Autodesk Inventor part; units mm, degrees
ref_plane "РабПлоскость2" through (-11.5, 28.8975, 52.6492) normal (0, 0, -1) x (0, 1, 0)
ref_plane "РабПлоскость3" through (-11.5, 28.8975, 52.6492) normal (0, 0, -1) x (0, 1, 0)
ref_plane "РабПлоскость4" through (-15, 28.8975, 52.6492) normal (0, -1, 0) x (1, 0, 0)
ref_plane "РабПлоскость1" through (0, 34.8975, 74.4992) normal (0, 0, -1) x (1, 0, 0)
sketch "Эскиз1" plane through (0, 34.8975, 74.4992) normal (0, 0, -1) x (1, 0, 0)
  line L0 (11.5, 6) -> (11.5, -6)
  line L1 (15, -6) -> (11.5, -6)
  arc A0 (15, -6) -> (16, -5) centre (15, -5) ccw
  line L2 (16, -1.25) -> (16, -5)
  line L3 (14, -1.25) -> (16, -1.25)
  arc A1 (12.8, -0.05) -> (14, -1.25) centre (14, -0.05) ccw
  line L4 (12.8, 0.05) -> (12.8, -0.05)
  arc A2 (14, 1.25) -> (12.8, 0.05) centre (14, 0.05) ccw
  line L5 (16, 1.25) -> (14, 1.25)
  line L6 (16, 5) -> (16, 1.25)
  arc A3 (16, 5) -> (15, 6) centre (15, 5) ccw
  line L7 (11.5, 6) -> (15, 6)
  circle A4 centre (13.75, 3.5) radius 1.25
  circle A5 centre (13.75, -3.5) radius 1.25
  line L8 (-11.5, -6) -> (-11.5, 6)
  line L9 (-15, 6) -> (-11.5, 6)
  arc A6 (-15, 6) -> (-16, 5) centre (-15, 5) ccw
  line L10 (-16, 1.3872) -> (-16, 5)
  line L11 (-14, 1.3872) -> (-16, 1.3872)
  arc A7 (-12.802, 0.1186) -> (-14, 1.3872) centre (-14, 0.1872) ccw
  line L12 (-12.802, 0.0186) -> (-12.802, 0.1186)
  arc A8 (-14, -1.25) -> (-12.802, 0.0186) centre (-14, -0.05) ccw
  line L13 (-16, -1.25) -> (-14, -1.25)
  line L14 (-16, -5) -> (-16, -1.25)
  arc A9 (-16, -5) -> (-15, -6) centre (-15, -5) ccw
  line L15 (-11.5, -6) -> (-15, -6)
  circle A10 centre (-13.75, 3.5) radius 1.25
  circle A11 centre (-13.75, -3.5) radius 1.25
  line L16 (16, 5) -> (16, 6)
  line L17 (16, 6) -> (15, 6)
  line L18 (-16, 5) -> (-16, 6)
  line L19 (-16, 6) -> (-15, 6)
  line L20 (16, -5) -> (16, -6)
  line L21 (16, -6) -> (15, -6)
  line L22 (-16, -5) -> (-16, -6)
  line L23 (-16, -6) -> (-15, -6)
  point P0 (0, 34.8975)
extrude "Выдавливание1" add sketch "Эскиз1" along normal blind 6
sketch "Эскиз3" plane through (11.5, 28.8975, 74.4992) normal (0, -1, 0) x (1, 0, 0)
  line L0 (-23, 0) -> (-23, -6)
  line L1 (-23, -6) -> (-23, 0)
  line L2 (-23, 0) -> (-27.5, 0)
  line L3 (0, -6) -> (-23, -6)
  line L4 (-23, -6) -> (-23, 0)
  line L5 (-23, 0) -> (0, 0)
  line L6 (-23, -6) -> (-27.5, -6)
  line L7 (-23, -6) -> (-27.5, -6)
  line L8 (-27.5, -6) -> (-27.5, 0)
  line L9 (0, 0) -> (4.5, 0)
  line L10 (0, -6) -> (0, 0)
  line L11 (4.5, 0) -> (4.5, -6)
  line L12 (4.5, -6) -> (0, -6)
  point P0 (-11.5, -74.4992)
  point P1 (4.5, 0)
extrude "Выдавливание2" add sketch "Эскиз3" along normal blind 30
ref_plane "РабПлоскость2" through (-11.5, 28.8975, 52.6492) normal (0, 0, -1) x (0, 1, 0)
ref_plane "РабПлоскость3" through (-11.5, 28.8975, 52.6492) normal (0, 0, -1) x (0, 1, 0)
ref_plane "РабПлоскость6" through (-16, 2.8975, 68.4992) normal (0, 1, 0) x (1, 0, 0)
ref_plane "РабПлоскость4" through (-15, 28.8975, 52.6492) normal (0, -1, 0) x (1, 0, 0)
ref_plane "РабПлоскость8" through (-16, 2.8975, 68.4992) normal (0, 1, 0) x (1, 0, 0)
ref_plane "РабПлоскость5" through (-16, 2.8975, 68.4992) normal (0, 1, 0) x (1, 0, 0)
ref_plane "РабПлоскость7" through (16, 28.8975, 74.4992) normal (1, 0, 0) x (0, 0, -1)
ref_plane "РабПлоскость9" through (16, 28.8975, 74.4992) normal (-1, 0, 0) x (0, 0, 1)
ref_plane "РабПлоскость10" through (-16, 28.8975, 74.4992) normal (-1, 0, 0) x (0, 0, 1)
sketch "Эскиз14" plane through (11.5, -1.1025, 74.4992) normal (0, -1, 0) x (1, 0, 0)
  circle A0 centre (-3.5, -11.925) radius 2
  circle A1 centre (-19.5, -11.925) radius 2
  circle A2 centre (-3.5, -11.925) radius 1.5
  circle A3 centre (-19.5, -11.925) radius 1.5
  point P0 (-11.5, -74.4992)
  dimension "d38" = 3
  dimension "d39" = 3
extrude "Выдавливание12" add sketch "Эскиз14" against normal blind 4
ref_plane "РабПлоскость14" through (18, 28.8975, 74.4992) normal (1, 0, 0) x (0, 0, -1)
sketch "Эскиз15" plane through (18, 28.8975, 74.4992) normal (1, 0, 0) x (0, 0, -1)
  line L0 (1.45, -3.75) -> (1.45, -63.75)
  line L1 (-2.55, -3.75) -> (1.45, -3.75)
  line L2 (-2.55, -3.75) -> (1.45, -3.75)
  line L3 (1.45, -3.75) -> (1.45, -34.5952)
  line L4 (1.45, -34.5952) -> (-2.55, -34.5952)
  line L5 (-2.55, -34.5952) -> (-2.55, -3.75)
  point P0 (74.4992, -28.8975)
extrude "Выдавливание13" cut sketch "Эскиз15" against normal blind 100
ref_plane "РабПлоскость13" through (16, 2.8975, 68.4992) normal (0, 1, 0) x (1, 0, 0)
ref_plane "РабПлоскость12" through (-18, 28.8975, 74.4992) normal (-1, 0, 0) x (0, 0, 1)
ref_plane "РабПлоскость11" through (16, 28.8975, 52.6492) normal (0, 0, -1) x (-1, 0, 0)
sketch "Эскиз18" plane through (16, 28.8975, 52.6492) normal (0, 0, -1) x (-1, 0, 0)
  circle A0 centre (4, -6.8) radius 1.5
  circle A1 centre (28, -6.8) radius 1.5
  point P0 (16, -28.8975)
extrude "Выдавливание16" cut sketch "Эскиз18" along normal mid plane 73
sketch "Эскиз19" plane through (0, 34.8975, 68.4992) normal (0, 0, -1) x (-1, 0, 0)
  line L0 (-16, -36) -> (16, -36)
  line L1 (16, -1.3872) -> (16, -36)
  line L2 (-16, -36) -> (16, -36)
  line L3 (16, -36) -> (16, -16)
  line L4 (16, -16) -> (-16, -16)
  line L5 (-16, -16) -> (-16, -36)
  point P0 (0, -34.8975)
  point P1 (11.5, -36)
  point P2 (16, -36)
  dimension "d57" = 20
extrude "Выдавливание17" cut sketch "Эскиз19" along normal mid plane 200
sketch "Эскиз13" plane through (-16, 28.8975, 74.4992) normal (-1, 0, 0) x (0, 0, 1)
  line L0 (-21.85, 12) -> (0, 12)
  line L1 (0, 12) -> (0, -10)
  line L2 (0, -10) -> (-21.85, -10)
  line L3 (-21.85, -10) -> (-21.85, 12)
  line L4 (0, 4.6128) -> (0, -3.75)
  point P0 (-74.4992, -28.8975)
  point P1 (0, 12)
  point P2 (-21.85, -30)
  dimension "d60" = 21.85
  dimension "d61" = 22
  dimension "d62" = 0
sketch "Эскиз10" plane through (16, 28.8975, 74.4992) normal (1, 0, 0) x (0, 0, -1)
  line L0 (0, 12) -> (21.85, 12)
  line L1 (21.85, 12) -> (21.85, -10)
  line L2 (21.85, -10) -> (0, -10)
  line L3 (0, -10) -> (0, 12)
  line L4 (0, 12) -> (6, 12)
  line L5 (0, 4.75) -> (0, -3.75)
  point P0 (74.4992, -28.8975)
  point P1 (21.85, -30)
  dimension "d63" = 21.85
  dimension "d64" = 22
  dimension "d65" = 0
  dimension "d66" = 0
extrude "Выдавливание18" add sketch "Эскиз13" along normal blind 2
extrude "Выдавливание19" add sketch "Эскиз10" along normal blind 2
sketch "Эскиз20" plane through (-16, 18.8975, 52.6492) normal (0, -1, 0) x (1, 0, 0)
  line L0 (32, 4) -> (0, 4)
  line L1 (0, 4) -> (0, 15.85)
  line L2 (0, 15.85) -> (32, 15.85)
  line L3 (32, 15.85) -> (32, 4)
  line L4 (0, 0) -> (0, 15.85)
  line L5 (32, 15.85) -> (0, 15.85)
  circle A0 centre (24, 9.925) radius 1.5
  circle A1 centre (8, 9.925) radius 1.5
  point P0 (16, -52.6492)
  dimension "d71" = 32
  dimension "d72" = 11.85
  dimension "d73" = 0
  dimension "d74" = 0
  dimension "d75" = 3
  dimension "d76" = 3
  dimension "d77" = 8
  dimension "d78" = 8
  dimension "d79" = 5.925
  dimension "d80" = 5.925
extrude "Выдавливание20" add sketch "Эскиз20" against normal blind 8.75
sketch "Эскиз21" plane through (16, 28.8975, 74.4992) normal (-1, 0, 0) x (0, 0, 1)
  line L0 (-21.85, 12) -> (-17.85, 12)
  line L1 (-17.85, 12) -> (-17.85, -10)
  line L2 (-17.85, -10) -> (-21.85, -10)
  line L3 (-21.85, -10) -> (-21.85, 12)
  line L4 (-17.85, -10) -> (-21.85, -10)
  line L5 (-17.85, -10) -> (-17.85, -1.25)
  point P0 (-74.4992, -28.8975)
  point P1 (-19.85, -10)
  dimension "d83" = 4
  dimension "d84" = 22
  dimension "d85" = 0
  dimension "d86" = 0
extrude "Выдавливание21" add sketch "Эскиз21" along normal blind 32.5
sketch "Эскиз22" plane through (-18, 18.8975, 52.6492) normal (0, 0, -1) x (-1, 0, 0)
  line L0 (-29.5, 10) -> (-29.5, 22)
  line L1 (-6.5, 22) -> (-6.5, 10)
  line L2 (-29.5, 10) -> (-6.5, 10)
  line L3 (-6.5, 10) -> (-6.5, 22)
  line L4 (-6.5, 22) -> (-29.5, 22)
  line L5 (-29.5, 22) -> (-29.5, 10)
  point P0 (-18, -18.8975)
extrude "Выдавливание22" cut sketch "Эскиз22" against normal blind 32.5
chamfer "Фаска1" distance 2 angle 45 2 edges at (6.5, 27.6475, 62.5742) (-9.5, 27.6475, 62.5742)
properties part number "держатель сервомоторчика"
Geometry: final body of the model. Coordinates: model frame, mm. A direction names the side the tool comes from. Round coordinates to 2 decimals unless told otherwise and drop trailing zeros. Write each loop counter-clockwise with the first axis right and the second up, starting at its lowest first coordinate (ties: lowest second). Pieces come first, ordered by that corner, then holes. Notation, with made-up numbers: M 40,-13.5 L 95,-13.5 A6 ccw 95,-2.5 Z; hole C -28.5,11.5 d11. An arc over 180 degrees is marked long. Answer in a Markdown table with one row per item. Add a question column.
(1) Cut plane A-A, the plane x = 8. Return the cut outline in (y, z).
(2) Cut plane B-B, the plane y = 29.75. Return the cut outline in (x, z).
(3) Ray query, L1, parallel to X at y = 35, z = 69; L2, parallel to X at y = 36.75, z = 70.5; L3, parallel to Z at x = -15, y = 31. Return the intervals inside material, ascending.
(4) Contact query for flat-ended pins moving along their axis: pin 1 (12 mm diameter, centred on x = 13.5, y = 37.5, fed in from +Z); pin 2 (8 mm diameter, centred on x = -3, z = 68, fed in from +Y); pin 3 (3.5 mm diameter, centred on x = 8, z = 65.5, fed in from +Y); pin 4 (0.9 mm diameter, centred on x = -12.5, y = 22, fed in from +Z). Output: stop coordinate, or through.
(5) Cut plane C-C, the plane x = 12. Return the cut outline in (y, z).
(6) Cut plane D-D, the plane y = 22.5. Return the cut outline in (x, z), then the cut area to 3 significant figures.
(7) Reachability of faces 1 (the face through (-1, 28, 68.499)), 2 (the face through (13.479, 30.177, 71.541)), 3 (the face through (-11.5, 35, 72)), 4 (the face through (16, 22, 74)) from +Z, -Z, +X, -X, +Y, -Y: full face, straight path, thin tool, end or side. Return the list, or none.
(8) Draft query along X for faces 5 (the face through (18, 30, 64)), 6 (the face through (7.8, 22.23, 64.06)). Return one class per face: pulls with the +X half, pulls with the -X half, needs draft (parallel to the pull), parting line crosses it, or undercut.
Established:
| question | item | result |
|---|---|---|
| 1 | outline | M 18.9,52.65 L 28.9,52.65 L 28.9,56.65 L 27.65,56.65 L 27.65,59.07 L 25.65,61.07 L 18.9,61.07 Z; M 18.9,64.07 L 25.65,64.07 L 27.65,66.07 L 27.65,68.5 L 28.9,68.5 L 28.9,74.5 L 25.15,74.5 L 25.15,73.05 L 18.9,73.05 Z |
| 2 | outline | M -18,52.65 L -11.5,52.65 L -11.5,56.65 L -16,56.65 L -16,68.5 L -11.5,68.5 L -11.5,74.5 L -18,74.5 Z; M 11.5,52.65 L 18,52.65 L 18,74.5 L 11.5,74.5 L 11.5,68.5 L 16,68.5 L 16,56.65 L 11.5,56.65 Z |
| 3 | L1 | -18 to -16, -12.8 to -11.5, 11.5 to 12.8, 16 to 18 |
| 3 | L2 | -18 to -11.5, 11.5 to 18 |
| 3 | L3 | 52.65 to 56.65, 68.5 to 74.5 |
| 4 | pin 1 | z = 74.5 |
| 4 | pin 2 | y = 28.9 |
| 4 | pin 3 | y = 27.65 |
| 4 | pin 4 | z = 68.5 |
| 5 | outline | M 18.9,52.65 L 40.9,52.65 L 40.9,56.65 L 27.65,56.65 L 27.65,68.5 L 40.9,68.5 L 40.9,74.5 L 25.15,74.5 L 25.15,73.05 L 23.6,73.05 L 23.6,68.5 L 20.6,68.5 L 20.6,73.05 L 18.9,73.05 Z |
| 6 | outline | M -18,52.65 L 18,52.65 L 18,74.5 L 16,74.5 L 16,73.05 L 13.44,73.05 L 13.44,68.5 L 10.56,68.5 L 10.56,73.05 L -10.56,73.05 L -10.56,68.5 L -13.44,68.5 L -13.44,73.05 L -16,73.05 L -16,74.5 L -18,74.5 Z; hole C -8,62.57 d3; hole C 8,62.57 d3 |
| 6 | area | 700 mm² |
| 7 | face 1 | +Y |
| 7 | face 2 | +Z |
| 7 | face 3 | +Z, -Z, +Y |
| 7 | face 4 | +Z, -Y |
| 8 | face 5 | pulls with the +X half |
| 8 | face 6 | undercut |
